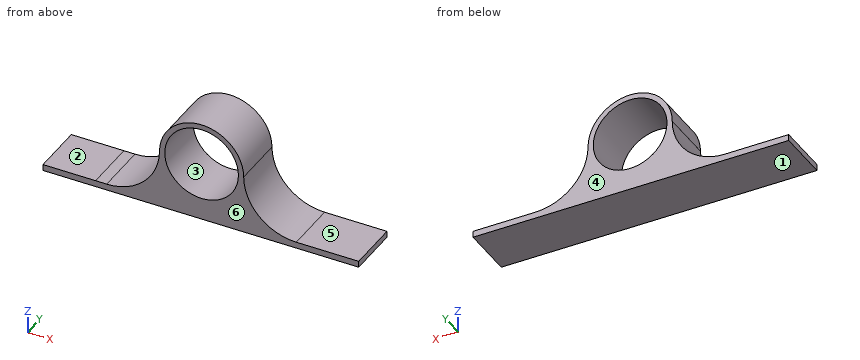
```python
from build123d import *

# Parameters (mm, degrees)
F0_R     = 17.5
F1_DEPTH = 25


# Not quite as in the source:
# - ends of sketch curves that miss each other by under 0.0002 mm in the source are joined


with BuildPart() as f1:
    # F0 (on Front) → F1 (new body)
    with BuildSketch(Plane.XZ):
        with BuildLine():
            ThreePointArc((45, -25), (27.3223304703, -17.6776695297), (20, 0))
            ThreePointArc((20, 0), (0.0107860663, -19.9999970915), (-19.9999883661, -0.0215721294))
            ThreePointArc((-19.9999883661, -0.0215721294), (-27.3583172251, -17.7351553161), (-45.1016823096, -25.0213653552))
            Line((-45.1016823096, -25.0213653552), (-50.3546064898, -25))
            Line((-50.3546064898, -25), (-75.3500018494, -25))
            Line((-75.3500018494, -25), (-75.3500018494, -28))
            Line((-75.3500018494, -28), (74.6500011308, -28))
            Line((74.6500011308, -28), (74.65, -25))
            Line((74.65, -25), (50.3546064898, -25))
            Line((50.3546064898, -25), (45, -25))
        make_face()
        with BuildLine():
            ThreePointArc((-19.9999883661, -0.0215721294), (0.0107860663, -19.9999970915), (20, 0))
            ThreePointArc((20, 0), (0, 20), (-20, 0))
            ThreePointArc((-20, 0), (-19.9999970915, -0.0107860663), (-19.9999883661, -0.0215721294))
        make_face()
        Circle(F0_R, mode=Mode.SUBTRACT)
    extrude(amount=F1_DEPTH)


solid = f1.part
```
Source: CAD feature listing. Evaluate the final solid. Frame: model axes, mm. Face numbers are marked on the shaded views. A direction names the side the tool comes from. Coordinates: 2 decimals unless noted, no trailing zeros. Order: outer loops, then holes, each group sorted by start corner. A loop starts at its lowest first (then second) coordinate and runs counter-clockwise, first axis right, second up. Notation, with made-up numbers: (-16.5, 16) - (-5.5, 16) arc R38 ccw to (-5.5, 55) - close; hole circle Ø9 at (-37, 51). An arc over 180 degrees is marked (long way). One line per item, written item: value.
1) Contact query for flat-ended pins moving along their axis: pin 1 (3 mm diameter, centred on y = -20, z = 3, fed in from +X); pin 2 (12.5 mm diameter, centred on x = -66.5, y = -8.5, fed in from +Z); pin 3 (4 mm diameter, centred on x = 5.5, z = 12.5, fed in from -Y); pin 4 (4 mm diameter, centred on y = -15.5, z = -9, fed in from -X). Output: stop coordinate, or through.
Computed values:
pin 1: stops at x = 19.94
pin 2: stops at z = -25
pin 3: passes through
pin 4: stops at x = -22.54
2) Cut plane D-D on x = -58. Output: boundary loops of the cut face in (y, z), plus the area to 3 significant figures.
Computed values:
outline: (-25, -28) - (0, -28) - (0, -25) - (-25, -25) - close
area: 75.0 mm^2
3) Mould query, pull axis Z, two halves, no side actions, for the marked faces 1, 2, 3 and 4. Classes: released by +Z, released by -Z, zero draft, split by the parting line, or undercut.
Computed values:
face 1: released by -Z
face 2: released by +Z
face 3: undercut
face 4: zero draft
4) Cut plane B-B on z = -9.5. Output: boundary loops of the cut face in (x, y), plus the area to 3 significant figures.
Computed values:
outline: (-21.87, -25) - (-14.7, -25) - (-14.7, 0) - (-21.87, 0) - close; (14.7, -25) - (21.88, -25) - (21.88, 0) - (14.7, 0) - close
area: 359 mm^2
5) Cut plane A-A on x = 0. Output: boundary loops of the cut face in (y, z), plus the area to 3 significant figures.
Computed values:
outline: (-25, -28) - (0, -28) - (0, -17.5) - (-25, -17.5) - close; (-25, 17.5) - (0, 17.5) - (0, 20) - (-25, 20) - close
area: 325 mm^2
6) Ray query, line 1 (Z direction, x = 0, y = -10); line 2 (X direction, y = -16, z = -7.5); line 3 (X direction, y = -13.5, z = 16). Return the intervals inside material, ascending. Write a range as [from, to].
Computed values:
line 1: z = [-28, -17.5], [17.5, 20]
line 2: x = [-21.14, -15.81], [15.81, 21.15]
line 3: x = [-12, -7.09], [7.09, 12]
7) Reachability of the marked faces 5 and 6 from +Z, -Z, +X, -X, +Y, -Y: full face, straight path, thin tool, end or side. Return the list, or none.
Computed values:
face 5: +Z, +X, +Y, -Y
face 6: +Z, -Z, +X, -X, -Y
